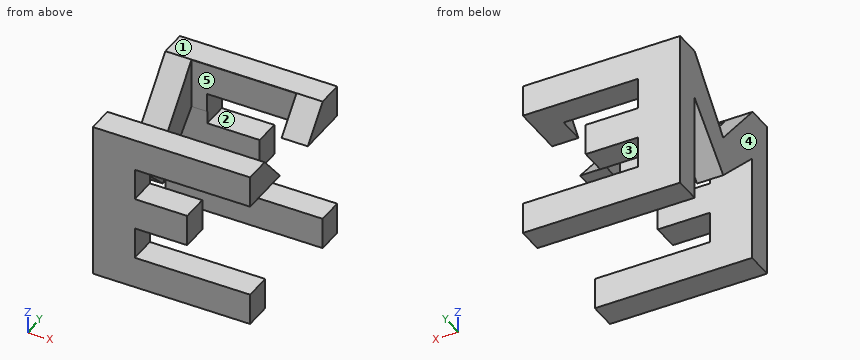
from build123d import *

# Parameters (mm, degrees)
F0_W      = 38.1
F0_H      = 38.1
F2_DEPTH  = 38.1
F4_DEPTH  = 38.1
F6_W      = 25.4
F6_H      = 24.634876
F8_DEPTH  = 38.1
F10_DEPTH = 38.1
F12_DEPTH = 38.1


with BuildPart() as f2:
    # F0 (on Front) → F2 (new body)
    with BuildSketch(Plane.XZ):
        with Locations((19.05, 19.05)):
            Rectangle(F0_W, F0_H)
    extrude(amount=F2_DEPTH)

    # F3 (on Front) → F4 (cut)
    with BuildSketch(Plane.XZ):
        Polygon((38.1, 7.62), (38.1, 30.48), (10.16, 30.48), (10.16, 22.86), (22.86, 22.86), (22.86, 15.24), (10.16, 15.24), (10.16, 7.62), align=None)
    extrude(amount=F4_DEPTH, mode=Mode.SUBTRACT)

    # F6 (on offset) → F8 (cut)
    with BuildSketch(Plane.XY.offset(38.1)):
        with Locations((19.05, -18.698502)):
            Rectangle(F6_W, F6_H)
    extrude(amount=-F8_DEPTH, mode=Mode.SUBTRACT)

    # F9 (on Right) → F10 (cut)
    with BuildSketch(Plane.YZ):
        Polygon((-18.861001, 23.382206), (-6.35, 38.1), (-31.735882, 38.1), align=None)
    extrude(amount=F10_DEPTH, mode=Mode.SUBTRACT)

    # F11 (on Right) → F12 (cut)
    with BuildSketch(Plane.YZ):
        Polygon((-31.504388, 0), (-6.35, 0), (-6.35, 25.959453), (-18.885972, 13.653007), (-31.504388, 25.785374), align=None)
    extrude(amount=F12_DEPTH, mode=Mode.SUBTRACT)


solid = f2.part
For this review, take the finished solid that the model builds, in its own axes (mm). Face numbers are marked on the shaded views. A direction names the side the tool comes from. Round coordinates to 2 decimals unless told otherwise and drop trailing zeros. Loops run counter-clockwise (first coordinate to the right, second up) from the corner with the lowest first, then second, coordinate; pieces in that order, holes last. Notation, with made-up numbers: (17.25, 79) - (22.25, 79) arc R20 cw to (22.25, 86) - close; hole circle Ø4 at (-1.75, 82). An arc over 180 degrees is marked (long way). Use one line per item in the form item = value.
Item 1: Mouldability with a two-part tool opening along X and no side actions: class the marked faces 3, 4 and 5 as +X half, -X half, draft (parallel to the pull), parting line (faces both ways), or undercut.
Answers:
face_3 = draft
face_4 = -X half
face_5 = undercut
Item 2: Tool access review of the marked faces 1 and 2: name each direction out of +Z, -Z, +X, -X, +Y, -Y from which nothing blocks a thin tool from reaching the whole face with its end or side.
Answers:
face_1 = +Z, +X, -X, +Y, -Y
face_2 = +X, +Y, -Y
Item 3: Consider section C-C on x = 14. Write out the cut boundary in (y, z).
Answers:
outline = (-38.1, 0) - (-31.5, 0) - (-31.5, 7.62) - (-38.1, 7.62) - close; (-38.1, 15.24) - (-31.5, 15.24) - (-31.5, 22.86) - (-38.1, 22.86) - close; (-38.1, 30.48) - (-31.02, 30.48) - (-31.02, 37.28) - (-31.74, 38.1) - (-38.1, 38.1) - close; (-6.38, 30.48) - (0, 30.48) - (0, 38.1) - (-6.35, 38.1) - (-6.38, 38.06) - close; (-6.35, 0) - (0, 0) - (0, 7.62) - (-6.35, 7.62) - close; (-6.35, 15.24) - (0, 15.24) - (0, 22.86) - (-6.35, 22.86) - close
Item 4: Clearance check with flat-ended pins moving along their axes: P1, Ø1.9, axis at y = -3, z = 10, coming from the +X side; P2, Ø2, axis at y = -36.5, z = 20, coming from the +X side; P3, Ø1, axis at y = -28, z = 27, coming from the +X side. State where each tip first meets the part, or that it passes through.
Answers:
P1 = 10.16
P2 = 22.86
P3 = 6.35
Item 5: Consider section B-B on z = 17.5. Write out the cut boundary in (x, y).
Answers:
outline = (0, -38.1) - (22.86, -38.1) - (22.86, -31.5) - (0, -31.5) - close; (0, -22.89) - (6.35, -22.89) - (6.35, -14.97) - (0, -14.97) - close; (0, -6.35) - (22.86, -6.35) - (22.86, 0) - (0, 0) - close
Item 6: Consider section A-A on x = 29. Write out the cut boundary in (y, z), then the cut area to 3 significant figures.
Answers:
outline = (-38.1, 0) - (-31.5, 0) - (-31.5, 7.62) - (-38.1, 7.62) - close; (-38.1, 30.48) - (-31.02, 30.48) - (-31.02, 37.28) - (-31.74, 38.1) - (-38.1, 38.1) - close; (-6.38, 30.48) - (0, 30.48) - (0, 38.1) - (-6.35, 38.1) - (-6.38, 38.06) - close; (-6.35, 0) - (0, 0) - (0, 7.62) - (-6.35, 7.62) - close
area = 201 mm^2
Item 7: For line 1 (Z direction, x = 14.5, y = -36); line 2 (X direction, y = -12, z = 31); line 3 (Y direction, x = 11.5, z = 33), list the stretches that pass through material, from the lowest coordinate up.
Answers:
line_1 = 0 to 7.62, 15.24 to 22.86, 30.48 to 38.1
line_2 = 0 to 6.35, 31.75 to 38.1
line_3 = -38.1 to -31.02, -6.38 to 0
Item 8: Consider section D-D on y = -4. Write out the cut boundary in (x, z).
Answers:
outline = (0, 0) - (38.1, 0) - (38.1, 7.62) - (10.16, 7.62) - (10.16, 15.24) - (22.86, 15.24) - (22.86, 22.86) - (10.16, 22.86) - (10.16, 30.48) - (38.1, 30.48) - (38.1, 38.1) - (0, 38.1) - close
